```python
from build123d import *

# Parameters (mm, degrees)
F0_R     = 5.385
F0_R_2   = 3.87
F1_DEPTH = 18.58
F2_R     = 5.385
F3_DEPTH = 0.47
F4_SIZE2 = 0.47
F4_SIZE  = 0.47
F5_R     = 4.405
F6_DEPTH = 1.14
F7_R     = 5.385
F8_DEPTH = 1.4
F9_SIZE2 = 0.3571058445
F9_SIZE  = 0.51


with BuildPart() as f1:
    # F0 (on Top) → F1 (new body)
    with BuildSketch(Plane.XY):
        Circle(F0_R)
        Circle(F0_R_2, mode=Mode.SUBTRACT)
    extrude(amount=F1_DEPTH)

    # F2 (on face) → F3 (join)
    with BuildSketch(Plane(origin=(0, 0, 0), x_dir=(1, 0, 0), z_dir=(0, 0, -1))):
        Circle(F2_R)
    extrude(amount=F3_DEPTH)

    # F4
    f4_edges = [f1.edges().sort_by_distance(p)[0] for p in [
        (-5.385, 0, -0.47),
    ]]
    chamfer(f4_edges, length=F4_SIZE, length2=F4_SIZE2)

    # F5 (on face) → F6 (join)
    with BuildSketch(Plane(origin=(0, 0, -0.47), x_dir=(1, 0, 0), z_dir=(0, 0, -1))):
        Circle(F5_R)
    extrude(amount=F6_DEPTH)

    # F7 (on face) → F8 (join)
    with BuildSketch(Plane(origin=(0, 0, -1.61), x_dir=(1, 0, 0), z_dir=(0, 0, -1))):
        Circle(F7_R)
    extrude(amount=F8_DEPTH)

    # F9
    f9_edges = [f1.edges().sort_by_distance(p)[0] for p in [
        (-5.385, 0, -3.01),
    ]]
    f9_side = f1.faces().sort_by_distance((0, 0, -3.01))[0]
    chamfer(f9_edges, length=F9_SIZE, length2=F9_SIZE2, reference=f9_side)


solid = f1.part
```
Part model, mm, in its own coordinate system. A direction names the side the tool comes from. Coordinates: 2 decimals unless noted, no trailing zeros. Write each loop counter-clockwise with the first axis right and the second up, starting at its lowest first coordinate (ties: lowest second). Pieces come first, ordered by that corner, then holes.
Item 1: Pin check, flat tips, straight feed: pin 1 (1.5 mm diameter, centred on x = -2, z = 13, fed in from +Y); pin 2 (1.5 mm diameter, centred on y = -1, z = 3.5, fed in from -X). Stop position of each tip, or through.
Item 2: Probe line 1 (Y direction, x = 0, z = 9.25) (3 decimals); line 2 (Z direction, x = 2, y = 4.25); line 3 (Z direction, x = -4.75, y = 2). List the from-to ranges inside material, lowest first.
Item 3: Mould opens along X. For faces 3 (the face through (-0.95, 4.3, -1.03)), 4 (the face through (0, 0, -3.01)), 5 (the face through (1.79, -3.43, 9.16)) say: released by +X, released by -X, zero draft, split by the parting line, or undercut.
Item 4: Which spindle directions (+Z, -Z, +X, -X, +Y, -Y) get a long thin tool onto all of the face, cutting with end or side? Do faces 1 (the face through (0, 0, 0)), 2 (the face through (-1, 4, 18.58)). Say none if no direction does.
Item 5: Slice it at C-C (z = 0.5). Write the cut outline in (x, y) (3 decimals), and give its area (3 significant figures).
Item 6: Slice it at A-A (y = 0). Write the cut outline in (x, z) (3 decimals), and give its area (3 significant figures).
Results found:
1. pin 1: stops at y = 5.24
1. pin 2: stops at x = -5.38
2. line 1: y = -5.385 to -3.87, 3.87 to 5.385
2. line 2: z = -3.01 to -1.61, -0.47 to 18.58
2. line 3: z = -2.81 to -1.61, -0.23 to 18.58
3. face 3: split by the parting line
3. face 4: zero draft
3. face 5: undercut
4. face 1: +Z
4. face 2: +Z, +X, -X, +Y, -Y
5. outline: circle Ø10.77 at (0, 0); hole circle Ø7.74 at (0, 0)
5. area: 44.0 mm2
6. outline: (-5.385, -2.653) - (-4.875, -3.01) - (4.875, -3.01) - (5.385, -2.653) - (5.385, -1.61) - (4.405, -1.61) - (4.405, -0.47) - (4.915, -0.47) - (5.385, 0) - (5.385, 18.58) - (3.87, 18.58) - (3.87, 0) - (-3.87, 0) - (-3.87, 18.58) - (-5.385, 18.58) - (-5.385, 0) - (-4.915, -0.47) - (-4.405, -0.47) - (-4.405, -1.61) - (-5.385, -1.61) - close
6. area: 86.1 mm2
